Input: part model. Units: mm. Frame: model coordinates. Coordinates: 2 decimals unless noted, no trailing zeros. Order: outer loops, then holes, each group sorted by start corner. A loop starts at its lowest first (then second) coordinate and runs counter-clockwise, first axis right, second up. Notation, with made-up numbers: (14.25, 15.25) - (65.25, 15.25) arc R17 ccw to (65.25, 36.25) - close; hole circle Ø11 at (47, 39). An arc over 180 degrees is marked (long way). One line per question, with ' | ' between items. Start each with the question number.
```python
from build123d import *

# Parameters (mm, degrees)
EXTRUDE1_DEPTH = 8.73125


with BuildPart() as part:
    # Sketch1 → Extrude1 (new body, symmetric)
    with BuildSketch(Plane.XY):
        with BuildLine():
            Line((-1.038085852, 0.183042544), (-0.587831748, 0.103650597))
            ThreePointArc((-0.587831748, 0.103650597), (0.5969, 0), (-0.587831748, -0.103650597))
            Line((-0.587831748, -0.103650597), (-1.038085852, -0.183042544))
            ThreePointArc((-1.038085852, -0.183042544), (1.0541, 0), (-1.038085852, 0.183042544))
        make_face()
    extrude(amount=EXTRUDE1_DEPTH, both=True)

    # Sketch2 → Cut-Revolve1 (revolve, cut)
    with BuildSketch(Plane(origin=(0, 0, 0), x_dir=(0, 0, -1), z_dir=(1, 0, 0))):
        Polygon((8.73125, 1.0541), (8.73125, 0.9525), (7.91845, 1.0541), align=None)
        Polygon((-7.91845, 1.0541), (-8.73125, 1.0541), (-8.73125, 0.9525), align=None)
    revolve(axis=Axis((0, 0, -8.73125), (0, 0, 1)), mode=Mode.SUBTRACT)


solid = part.part
```
(1) Material intervals for line 1 along Y through (x, z) = (0, 3.75); line 2 along X through (y, z) = (-0.4, -4.25); line 3 along X through (y, z) = (0, 0.5), sorted ascending. Write a range as from..to.
(2) Section B-B (z = 3). Output: boundary loops of the cut face in (x, y).
(3) Draft query along Y for faces 1 (the face through (1.053, -0.044, 0.111)), 2 (the face through (0.596, 0.025, 0.122)). Return one class per face: +Y half, -Y half, draft (parallel to the pull), parting line (faces both ways), or undercut.
(4) Section A-A (x = 0). Output: boundary loops of the cut face in (y, z), then the cut area to 3 significant figures.
Worked answers:
1) line 1: y = -1.05..-0.6, 0.6..1.05 | line 2: x = -0.98..-0.44, 0.44..0.98 | line 3: x = 0.6..1.05
2) outline: (-1.04, -0.18) arc R1.05 ccw (long way) to (-1.04, 0.18) - (-0.59, 0.1) arc R0.6 cw (long way) to (-0.59, -0.1) - close
3) face 1: parting line | face 2: undercut
4) outline: (-1.05, -7.92) - (-0.95, -8.73) - (-0.6, -8.73) - (-0.6, 8.73) - (-0.95, 8.73) - (-1.05, 7.92) - close; (0.6, -8.73) - (0.95, -8.73) - (1.05, -7.92) - (1.05, 7.92) - (0.95, 8.73) - (0.6, 8.73) - close | area: 15.8 mm²
